Geometry: final body of the model. Coordinates: model frame, mm. A direction names the side the tool comes from. Coordinates: 2 decimals unless noted, no trailing zeros. Order: outer loops, then holes, each group sorted by start corner. A loop starts at its lowest first (then second) coordinate and runs counter-clockwise, first axis right, second up. Notation, with made-up numbers: (-25.75, -12) -> (-21.75, -12) arc R25 ccw to (-21.75, 11) -> close; hole circle Ø8 at (64.25, -12.5). An arc over 180 degrees is marked (long way). Answer in a Markdown table with one row per item. Add a question column.
1) Contact query for flat-ended pins moving along their axis: P1, Ø2, axis at x = -58.5, z = 269, coming from the +Y side; P2, Ø6, axis at x = -175.5, y = 3, coming from the +Z side; P3, Ø3, axis at x = 117.5, z = 446, coming from the +Y side; P4, Ø2, axis at x = -135, y = -150, coming from the +Z side. Output: stop coordinate, or through.
2) Section query A-A on z = 321. Return the cut outline in (x, y), then the cut area to 3 significant figures.
3) Set-up query: faces 4 (the face through (175, 0, 13)), 5 (the face through (-2, 2, 15)), 6 (the face through (4, -168, 5)), 7 (the face through (0, -175, 13)). Return all of +Z, -Z, +X, -X, +Y, -Y with unobstructed straight access to the full face (end or side cutting, diameter ignored); none if empty.
4) Section query B-B on y = -158.5. Return the cut outline in (x, z), then the cut area to 3 significant figures.
5) Ray query, line 1 (Y direction, x = 0, z = 8.25); line 2 (Y direction, x = 0, z = 423); line 3 (Z direction, x = 85.5, y = 78.5). Return the intervals inside material, ascending. Write a range as from..to.
6) Pull-direction query (Y, two-part tool) for faces 1 (the face through (-111.1, -85.19, 256.64)), 2 (the face through (-2, 2, 500)), 3 (the face through (-2, 2, 485)); classes: +Y half, -Y half, draft (parallel to the pull), parting line (faces both ways), or undercut.
```python
from build123d import *

# Parameters (mm, degrees)
SKIZZE1_R                       = 200
AUFSATZ_LINEAR_AUSTRAGEN1_DEPTH = 10
SKIZZE2_R                       = 140
AUFSATZ_LINEAR_AUSTRAGEN2_DEPTH = 490
VERRUNDUNG2_R                   = 10
SKIZZE8_R                       = 10
SCHNITT_LINEAR_AUSTRAGEN1_DEPTH = 5
AUFSATZ_LINEAR_AUSTRAGEN4_DEPTH = 8
WANDUNG1_T                      = 15


with BuildPart() as part:
    # Skizze1 → Aufsatz-Linear austragen1 (new body)
    with BuildSketch(Plane.XY):
        Circle(SKIZZE1_R)
    extrude(amount=AUFSATZ_LINEAR_AUSTRAGEN1_DEPTH)

    # Skizze2 → Aufsatz-Linear austragen2 (add)
    with BuildSketch(Plane.XY.offset(10)):
        Circle(SKIZZE2_R)
    extrude(amount=AUFSATZ_LINEAR_AUSTRAGEN2_DEPTH)

    # Verrundung2
    verrundung2_edges = [part.edges().sort_by_distance(p)[0] for p in [
        (-140, 0, 10),
    ]]
    fillet(verrundung2_edges, radius=VERRUNDUNG2_R)

    # Skizze8 → Schnitt-Linear austragen1 (cut)
    with BuildSketch(Plane.XY.offset(10)):
        with Locations((0, 175)):
            Circle(SKIZZE8_R)
        with Locations((175, 0)):
            Circle(SKIZZE8_R)
        with Locations((0, -175)):
            Circle(SKIZZE8_R)
        with Locations((-175, 0)):
            Circle(SKIZZE8_R)
    extrude(amount=-SCHNITT_LINEAR_AUSTRAGEN1_DEPTH, mode=Mode.SUBTRACT)

    # Skizze9 → Aufsatz-Linear austragen4 (add)
    with BuildSketch(Plane.XY.offset(5)):
        Polygon((0, 166.339745962), (7.5, 170.669872981), (7.5, 179.330127019), (0, 183.660254038), (-7.5, 179.330127019), (-7.5, 170.669872981), align=None)
        Polygon((-166.339745962, 0), (-170.669872981, 7.5), (-179.330127019, 7.5), (-183.660254038, 0), (-179.330127019, -7.5), (-170.669872981, -7.5), align=None)
        Polygon((166.339745962, 0), (170.669872981, -7.5), (179.330127019, -7.5), (183.660254038, 0), (179.330127019, 7.5), (170.669872981, 7.5), align=None)
        Polygon((0, -166.339745962), (-7.5, -170.669872981), (-7.5, -179.330127019), (0, -183.660254038), (7.5, -179.330127019), (7.5, -170.669872981), align=None)
    extrude(amount=AUFSATZ_LINEAR_AUSTRAGEN4_DEPTH)

    # Wandung1 (no face opened: a closed hollow body)
    add(offset(amount=-WANDUNG1_T, mode=Mode.PRIVATE), mode=Mode.SUBTRACT)


solid = part.part
```
Result:
| question | item | result |
|---|---|---|
| 1 | P1 | y = 127.65 |
| 1 | P2 | z = 13 |
| 1 | P3 | y = 78.38 |
| 1 | P4 | through |
| 2 | outline | circle Ø280 at (0, 0); hole circle Ø250 at (0, 0) |
| 2 | area | 12,500 mm2 |
| 3 | face 4 | +Z, +X, +Y, -Y |
| 3 | face 5 | none |
| 3 | face 6 | +Z |
| 3 | face 7 | +Z, +X, -X, -Y |
| 4 | outline | (-121.97, 0) -> (121.97, 0) -> (121.97, 10) -> (-121.97, 10) -> close |
| 4 | area | 2,440 mm2 |
| 5 | line 1 | -200..-185, -183.66..-166.34, -165..165, 166.34..183.66, 185..200 |
| 5 | line 2 | -140..-125, 125..140 |
| 5 | line 3 | 0..15, 485..500 |
| 6 | face 1 | parting line |
| 6 | face 2 | draft |
| 6 | face 3 | undercut |
